The listing builds one solid part. Answer for the finished solid, in the listing's coordinates (mm). A direction names the side the tool comes from. Give positions to 0.01 mm unless a question says otherwise; leave off trailing zeros. Loops run counter-clockwise (first coordinate to the right, second up) from the corner with the lowest first, then second, coordinate; pieces in that order, holes last. Notation, with made-up numbers: M 45,-39 L 96,-39 A17 ccw 96,-20 Z; hole C 14,87 d11. An arc over 180 degrees is marked long. One line per item, written item: value. Start each with the question number.
Q1. A cutting plane is placed at D-D, the plane z = 23. Determine the outline of the cut face in (x, y).
Q2. A cutting plane is placed at A-A, the plane z = 11. Determine the outline of the cut face in (x, y).
Q3. The mould has two halves that part along Y. Classify faces 1 (the cylindrical face through (11.075, 115.314, 0.986)), 2 (the cylindrical face through (9.675, 0.986, 33.536)), 3 (the flat face through (19, 0, 22)): +Y half, -Y half, draft (parallel to the pull), parting line (faces both ways), or undercut.
Q4. A cutting plane is placed at C-C, the plane y = 9. Determine the outline of the cut face in (x, z).
Q5. Consider L1, parallel to Y at x = 10, z = 1.25; L2, parallel to Z at x = 10, y = 0.9; L3, parallel to Z at x = 6, y = 108. Determine where each line is inside the solid, lowest interval first.
Q6. Flat-ended cylindrical pins translate along their axes: pin 1 (1.2 mm diameter, centred on x = 5, y = 114, fed in from -Z); pin 2 (2 mm diameter, centred on x = 3, z = 44, fed in from +Y); pin 3 (16.5 mm diameter, centred on y = 6.5, z = 20, fed in from -X); pin 4 (2.5 mm diameter, centred on x = 10, y = 110, fed in from -Z). Find the tip coordinate at first contact, or state that the pin passes through.
Q7. A cutting plane is placed at B-B, the plane x = 37.5. Determine the outline of the cut face in (y, z).
Q8. For faces 4 (the flat face through (0, 72, 1)), 5 (the flat face through (17, 64, 3)), 6 (the flat face through (9.5, 116.5, 2)), 7 (the cylindrical face through (18.345, 65.978, 43.986)), determine the directions among +Z, -Z, +X, -X, +Y, -Y from which every point of the face is accessible in a straight line to the end or side of a thin tool.
from build123d import *

# Parameters (mm, degrees)
SKETCH_R        = 2
SKETCH_R_2      = 0.5
PAD_DEPTH       = 3
SKETCH003_R     = 2
POCKET_DEPTH    = 2
PAD001_DEPTH    = 40
SKETCH001_R     = 4
PAD002_DEPTH    = 2
SKETCH004_R     = 6
SKETCH004_R_2   = 1.5
POCKET001_DEPTH = 5
SKETCH005_R     = 4
POCKET002_DEPTH = 1.5


with BuildPart() as part:
    # Sketch → Pad (new body)
    with BuildSketch(Plane.XY):
        with BuildLine():
            Line((0, 0), (30.712315, 0))
            ThreePointArc((30.712315, 0), (41.547219, 60), (30.712315, 120))
            Line((21.18034, 120), (30.712315, 120))
            ThreePointArc((21.18034, 120), (-0.606602, 120.606602), (0, 98.81966))
            Line((0, 98.81966), (0, 45))
            Line((10, 45), (0, 45))
            ThreePointArc((10, 15), (25, 30), (10, 45))
            Line((10, 15), (0, 15))
            Line((0, 15), (0, 0))
        make_face()
        with Locations((10, 110)):
            Circle(SKETCH_R, mode=Mode.SUBTRACT)
        with Locations((10, 117)):
            Circle(SKETCH_R_2, mode=Mode.SUBTRACT)
        with Locations((17, 110)):
            Circle(SKETCH_R_2, mode=Mode.SUBTRACT)
        with Locations((10, 103)):
            Circle(SKETCH_R_2, mode=Mode.SUBTRACT)
        with Locations((3, 110)):
            Circle(SKETCH_R_2, mode=Mode.SUBTRACT)
        with Locations((14.949747, 114.949747)):
            Circle(SKETCH_R_2, mode=Mode.SUBTRACT)
        with Locations((14.949747, 105.050253)):
            Circle(SKETCH_R_2, mode=Mode.SUBTRACT)
        with Locations((5.050253, 105.050253)):
            Circle(SKETCH_R_2, mode=Mode.SUBTRACT)
        with Locations((5.050253, 114.949747)):
            Circle(SKETCH_R_2, mode=Mode.SUBTRACT)
    extrude(amount=PAD_DEPTH)

    # Sketch003 → Pocket (cut)
    with BuildSketch(Plane(origin=(0, 0, 0), x_dir=(1, 0, 0), z_dir=(0, 0, -1))):
        with Locations((5.050253, -114.949747)):
            Circle(SKETCH003_R)
        with Locations((5.050253, -105.050253)):
            Circle(SKETCH003_R)
        with Locations((14.949747, -105.050253)):
            Circle(SKETCH003_R)
        with Locations((14.949747, -114.949747)):
            Circle(SKETCH003_R)
        with Locations((10, -103)):
            Circle(SKETCH003_R)
        with Locations((17, -110)):
            Circle(SKETCH003_R)
        with Locations((10, -117)):
            Circle(SKETCH003_R)
        with Locations((3, -110)):
            Circle(SKETCH003_R)
    extrude(amount=-POCKET_DEPTH, mode=Mode.SUBTRACT)

    # Sketch002 (on Face20 of Pad) → Pad001 (join)
    with BuildSketch(Plane.XY.offset(3)):
        with BuildLine():
            ThreePointArc((30.712315, 0), (41.547219, 60), (30.712315, 120))
            Line((30.712315, 120), (27.712315, 120))
            ThreePointArc((27.712315, 2), (39.40543, 61), (27.712315, 120))
            Line((0, 2), (27.712315, 2))
            Line((0, 0), (0, 2))
            Line((30.712315, 0), (0, 0))
        make_face()
    extrude(amount=PAD001_DEPTH)

    # Sketch001 (on Face33 of Pad001) → Pad002 (join)
    with BuildSketch(Plane.XY.offset(43)):
        with BuildLine():
            Line((10, 15), (0, 15))
            Line((0, 15), (0, 0))
            Line((0, 0), (30.712315, 0))
            ThreePointArc((30.712315, 0), (41.547219, 60), (30.712315, 120))
            Line((30.712315, 120), (21.18034, 120))
            ThreePointArc((21.18034, 120), (-0.606586, 120.606617), (-3.3e-05, 98.81969))
            ThreePointArc((25, 30), (18.168448, 66.46902), (-3.3e-05, 98.81969))
            ThreePointArc((10, 15), (20.606602, 19.393398), (25, 30))
        make_face()
        with Locations((10, 110)):
            Circle(SKETCH001_R, mode=Mode.SUBTRACT)
    extrude(amount=PAD002_DEPTH)

    # Sketch004 (on Face32 of Pad002) → Pocket001 (cut)
    with BuildSketch(Plane.XZ):
        with Locations((10, 23)):
            Circle(SKETCH004_R)
        with Locations((10, 35)):
            Circle(SKETCH004_R_2)
        with Locations((10, 11)):
            Circle(SKETCH004_R_2)
    extrude(amount=-POCKET001_DEPTH, mode=Mode.SUBTRACT)

    # Sketch005 (on Face4 of Pocket001) → Pocket002 (cut)
    with BuildSketch(Plane(origin=(0, 0, 0), x_dir=(1, 0, 0), z_dir=(0, 0, -1))):
        with Locations((10, -110)):
            Circle(SKETCH005_R)
    extrude(amount=-POCKET002_DEPTH, mode=Mode.SUBTRACT)


solid = part.part
Answer block:
1. outline: M 0,0 L 4,0 L 4,2 L 0,2 Z; M 16,0 L 30.71,0 A171.55 ccw 30.71,120 L 27.71,120 A154.69 cw 27.71,2 L 16,2 Z
2. outline: M 0,0 L 8.5,0 L 8.5,2 L 0,2 Z; M 11.5,0 L 30.71,0 A171.55 ccw 30.71,120 L 27.71,120 A154.69 cw 27.71,2 L 11.5,2 Z
3. face 1: undercut
3. face 2: draft
3. face 3: -Y half
4. outline: M 0,0 L 33.79,0 L 33.79,45 L 0,45 L 0,43 L 30.4,43 L 30.4,3 L 0,3 Z
5. L1: 0 to 15, 45 to 101, 105 to 106, 114 to 115, 119 to 125
5. L2: 0 to 9.5, 12.5 to 17, 29 to 33.5, 36.5 to 45
5. L3: 0 to 3, 43 to 45
6. pin 1: z = 2
6. pin 2: y = 123.75
6. pin 3: x = 0
6. pin 4: through
7. outline: M 22.96,0 L 97.04,0 L 97.04,45 L 22.96,45 Z; hole M 36.79,3 L 85.21,3 L 85.21,43 L 36.79,43 Z
8. face 4: +Z, -Z, -X, -Y
8. face 5: -X
8. face 6: -Z
8. face 7: +Z, -X
